Source: CAD feature listing. Evaluate the final solid. Frame: model axes, mm. A direction names the side the tool comes from. Round coordinates to 2 decimals unless told otherwise and drop trailing zeros. Write each loop counter-clockwise with the first axis right and the second up, starting at its lowest first coordinate (ties: lowest second). Pieces come first, ordered by that corner, then holes.
from build123d import *

# Parameters (mm, degrees)
SKETCH1_W           = 75
SKETCH1_H           = 18
BOSS_EXTRUDE1_DEPTH = 57
SKETCH1_3_R         = 3
BOSS_EXTRUDE2_DEPTH = 20
BOSS_EXTRUDE3_START = -18
SKETCH2_R           = 8.5
SKETCH2_R_2         = 3
BOSS_EXTRUDE3_DEPTH = 10
SKETCH2_2_R         = 3
CUT_EXTRUDE3_DEPTH  = 18
SKETCH3_W           = 10
SKETCH3_H           = 5
CUT_EXTRUDE4_DEPTH  = 10


with BuildPart() as part:
    # Sketch1 → Boss-Extrude1 (new body)
    with BuildSketch(Plane.XY):
        with Locations((37.5, -9)):
            Rectangle(SKETCH1_W, SKETCH1_H)
        Polygon((19.132863896, -10.6), (23.867136104, -10.6), (26.234272207, -6.5), (23.867136104, -2.4), (19.132863896, -2.4), (16.765727793, -6.5), align=None, mode=Mode.SUBTRACT)
        Polygon((58.234272207, -6.5), (55.867136104, -10.6), (51.132863896, -10.6), (48.765727793, -6.5), (51.132863896, -2.4), (55.867136104, -2.4), align=None, mode=Mode.SUBTRACT)
    extrude(amount=BOSS_EXTRUDE1_DEPTH)

    # Sketch1<3> → Boss-Extrude2 (add)
    # profile 1 of 2: a face of its own
    with BuildSketch(Plane.XY):
        Polygon((16.765727793, -6.5), (19.132863896, -10.6), (23.867136104, -10.6), (26.234272207, -6.5), (23.867136104, -2.4), (19.132863896, -2.4), align=None)
        with Locations((21.5, -6.5)):
            Circle(SKETCH1_3_R, mode=Mode.SUBTRACT)
    # profile 2 of 2: a face of its own
    with BuildSketch(Plane.XY):
        Polygon((55.867136104, -10.6), (58.234272207, -6.5), (55.867136104, -2.4), (51.132863896, -2.4), (48.765727793, -6.5), (51.132863896, -10.6), align=None)
        with Locations((53.5, -6.5)):
            Circle(SKETCH1_3_R, mode=Mode.SUBTRACT)
    extrude(amount=BOSS_EXTRUDE2_DEPTH)

    # Sketch2 → Boss-Extrude3 (add)
    # profile 1 of 2: a face of its own
    with BuildSketch(Plane(origin=(0, 0, 0), x_dir=(1, 0, 0), z_dir=(0, 1, 0)).offset(BOSS_EXTRUDE3_START)):
        with Locations(Location((12.5, -38.99, 0), (0, 0, 270))):
            Circle(SKETCH2_R)
        with Locations(Location((12.5, -38.99, 0), (0, 0, 270))):
            Circle(SKETCH2_R_2, mode=Mode.SUBTRACT)
    # profile 2 of 2: a face of its own
    with BuildSketch(Plane(origin=(0, 0, 0), x_dir=(1, 0, 0), z_dir=(0, 1, 0)).offset(BOSS_EXTRUDE3_START)):
        with Locations(Location((62.5, -38.99, 0), (0, 0, 270))):
            Circle(SKETCH2_R)
        with Locations(Location((62.5, -38.99, 0), (0, 0, 270))):
            Circle(SKETCH2_R_2, mode=Mode.SUBTRACT)
    extrude(amount=-BOSS_EXTRUDE3_DEPTH)

    # Sketch2<2> → Cut-Extrude3 (cut)
    with BuildSketch(Plane(origin=(0, 0, 0), x_dir=(1, 0, 0), z_dir=(0, 1, 0))):
        with Locations(Location((12.5, -38.99, 0), (0, 0, 270))):
            Circle(SKETCH2_2_R)
        with Locations(Location((62.5, -38.99, 0), (0, 0, 270))):
            Circle(SKETCH2_2_R)
    extrude(amount=-CUT_EXTRUDE3_DEPTH, mode=Mode.SUBTRACT)

    # Sketch3 → Cut-Extrude4 (cut)
    with BuildSketch(Plane.XZ.offset(18)):
        with Locations((21.5, 22)):
            Rectangle(SKETCH3_W, SKETCH3_H)
        with Locations((53.5, 22)):
            Rectangle(SKETCH3_W, SKETCH3_H)
    extrude(amount=-CUT_EXTRUDE4_DEPTH, mode=Mode.SUBTRACT)


solid = part.part
1) Pull-direction query (Z, two-part tool) for faces 4 (the face through (57.328, -22.93, 32.245)), 5 (the face through (21, -3, 20)), 6 (the face through (49, -8, 22)), 7 (the face through (57.034, -4.421, 38.241)); classes: released by +Z, released by -Z, zero draft, split by the parting line, or undercut.
Taken from the geometry:
face 4: split by the parting line
face 5: released by +Z
face 6: undercut
face 7: zero draft
2) Material intervals for line 1 (X direction, y = -6.5, z = 6.25); line 2 (X direction, y = -6.5, z = 38.99); line 3 (Y direction, x = 24.5, z = 35), sorted ascending.
Taken from the geometry:
line 1: x = 0 to 18.5, 24.5 to 50.5, 56.5 to 75
line 2: x = 0 to 9.5, 15.5 to 16.77, 26.23 to 48.77, 58.23 to 59.5, 65.5 to 75
line 3: y = -18 to -9.5, -3.5 to 0
3) Reachability of faces 1 (the face through (50.5, -6.4, 9.9)), 2 (the face through (26, -8, 22)), 3 (the face through (54, -10.6, 41)) from +Z, -Z, +X, -X, +Y, -Y: full face, straight path, thin tool, end or side. Return the list, or none.
Taken from the geometry:
face 1: +Z, -Z
face 2: -Y
face 3: +Z
4) Section query C-C on x = 62.5. Return the cut outline in (y, z).
Taken from the geometry:
outline: (-28, 30.49) - (-18, 30.49) - (-18, 0) - (0, 0) - (0, 35.99) - (-28, 35.99) - close; (-28, 41.99) - (0, 41.99) - (0, 57) - (-18, 57) - (-18, 47.49) - (-28, 47.49) - close
5) Section query A-A on z = 38.99. State how many separate pieces and enclosed holes the cut face has, then the cut area to 3 significant figures.
Taken from the geometry:
separate pieces: 3
enclosed holes: 2
area: 1,240 mm2
6) Contact query for flat-ended pins moving along their axis: P1, Ø12, axis at y = -20.5, z = 47.5, coming from the -X side; P2, Ø1, axis at y = -24.5, z = 28.5, coming from the +X side; P3, Ø1.2, axis at x = 50, z = 22.5, coming from the -Y side; P4, Ø1.5, axis at x = 31, z = 11, coming from the -Y side. Output: stop coordinate, or through.
Taken from the geometry:
P1: stops at x = 0
P2: passes through
P3: stops at y = -8
P4: stops at y = -18
7) Section query B-B on z = 52. Return the cut outline in (x, y).
Taken from the geometry:
outline: (0, -18) - (75, -18) - (75, 0) - (0, 0) - close; hole (16.77, -6.5) - (19.13, -10.6) - (23.87, -10.6) - (26.23, -6.5) - (23.87, -2.4) - (19.13, -2.4) - close; hole (48.77, -6.5) - (51.13, -10.6) - (55.87, -10.6) - (58.23, -6.5) - (55.87, -2.4) - (51.13, -2.4) - close
8) Section query D-D on y = -23.5. Return the cut outline in (x, z), then the cut area to 3 significant figures.
Taken from the geometry:
outline: circle Ø17 at (12.5, 38.99); circle Ø17 at (62.5, 38.99); hole circle Ø6 at (12.5, 38.99); hole circle Ø6 at (62.5, 38.99)
area: 397 mm2
